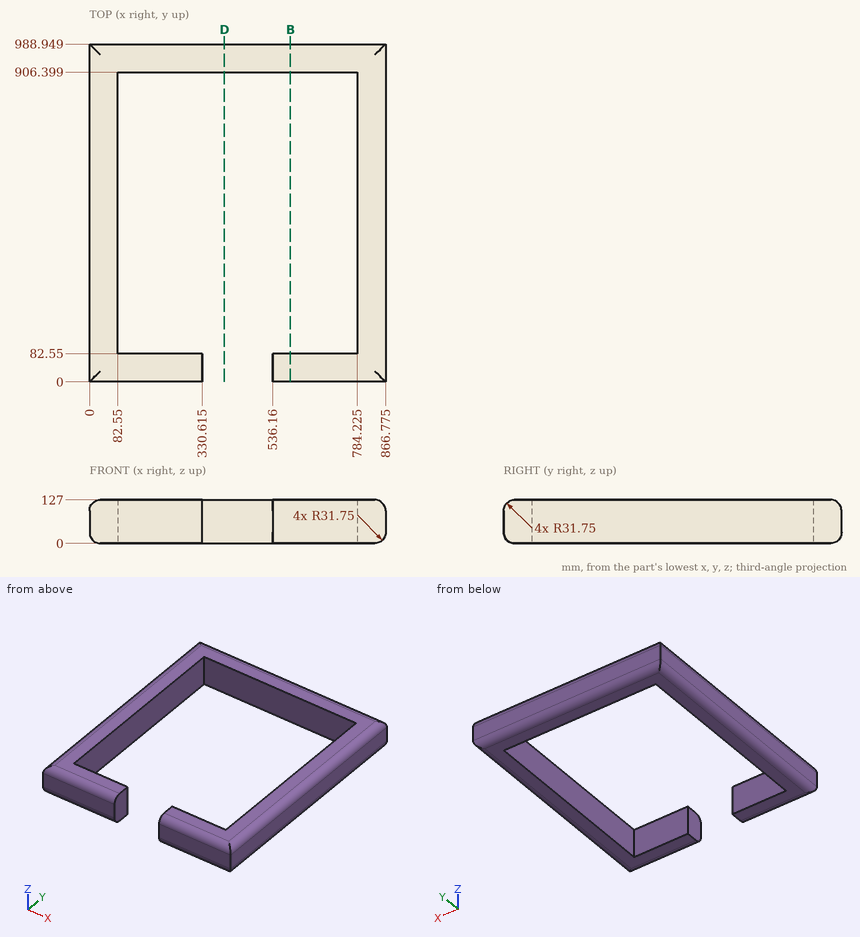
Source: three-view drawing plus pictorial views. Frame: mm from the lowest corner of the part. Coordinates: 2 decimals unless noted, no trailing zeros. Loops run counter-clockwise (first coordinate to the right, second up) from the corner with the lowest first, then second, coordinate; pieces in that order, holes last. Notation, with made-up numbers: (37.5, 22.25) - (51.5, 22.25) arc R35 cw to (51.5, 58.25) - close; hole circle Ø10 at (-8.5, 32). An arc over 180 degrees is marked (long way). One line per question, with ' | ' between items.
1) Section D-D, the plane x = 394.5. Return loops of the section in (y, z), then the cut area to 3 significant figures.
Report:
outline: (906.4, 0) - (957.2, 0) arc R31.75 ccw to (988.95, 31.75) - (988.95, 95.25) arc R31.75 ccw to (957.2, 127) - (906.4, 127) - close | area: 10,100 mm²
2) Section B-B, the plane x = 588. Return loops of the section in (y, z), then the cut area to 3 significant figures.
Report:
outline: (0, 31.75) arc R31.75 ccw to (31.75, 0) - (82.55, 0) - (82.55, 127) - (31.75, 127) arc R31.75 ccw to (0, 95.25) - close; (906.4, 0) - (957.2, 0) arc R31.75 ccw to (988.95, 31.75) - (988.95, 95.25) arc R31.75 ccw to (957.2, 127) - (906.4, 127) - close | area: 20,100 mm²
3) First-contact query: P1, Ø10, axis at x = 542.5, z = 26.5, coming from the -Y side. Flat tip, straight axial feed; report the tip coordinate or a pass-through.
Report:
P1: stops at y = 0
4) Line query: line 1 along Y through (x, z) = (580, 60.5); line 2 along Y through (x, z) = (456.5, 85.5); line 3 along Y through (x, z) = (530.5, 106). Output: solid intervals per line, ascending.
Report:
line 1: y = 0 to 82.55, 906.4 to 988.95 | line 2: y = 906.4 to 988.95 | line 3: y = 906.4 to 987.07
